from build123d import *

# Parameters (mm, degrees)
PAD029_DEPTH         = 16
SKETCH091_R          = 2.5
POCKET046_DEPTH      = 42.001
SKETCH092_R          = 2.63
POCKET047_DEPTH      = 30.001
POCKET047_DEPTH_BACK = 0.001


with BuildPart() as part:
    # Sketch089 → Pad029 (new body)
    with BuildSketch(Plane.XZ.offset(37.4)):
        with BuildLine():
            Line((-13, 31), (-10.5, 31))
            Line((-10.5, 10.5), (-10.5, 31))
            Line((10.5, 10.5), (-10.5, 10.5))
            Line((10.5, 31), (10.5, 10.5))
            Line((10.5, 31), (13, 31))
            ThreePointArc((15, 29), (14.414214, 30.414214), (13, 31))
            Line((15, 29), (15, 5.5))
            Line((15, 5.5), (13, 3.5))
            Line((13, 3.5), (13, -3.5))
            Line((13, -3.5), (15, -5.5))
            Line((15, -5.5), (15, -11))
            Line((15, -11), (-15, -11))
            Line((-15, -11), (-15, -5.5))
            Line((-13, -3.5), (-15, -5.5))
            Line((-13, 3.5), (-13, -3.5))
            Line((-15, 5.5), (-13, 3.5))
            Line((-15, 5.5), (-15, 29))
            ThreePointArc((-13, 31), (-14.414214, 30.414214), (-15, 29))
        make_face()
    extrude(amount=-PAD029_DEPTH)

    # Sketch091 → Pocket046 (cut, through all)
    with BuildSketch(Plane(origin=(0, 0, -11), x_dir=(-1, 0, 0), z_dir=(0, 0, -1))):
        with Locations((0, -29)):
            Circle(SKETCH091_R)
    extrude(amount=-POCKET046_DEPTH, mode=Mode.SUBTRACT)

    # Sketch092 → Pocket047 (cut, two sides)
    with BuildSketch(Plane(origin=(15, -29.4, 0), x_dir=(0, 1, 0), z_dir=(1, 0, 0))) as pocket047_sk:
        with Locations((0, 22)):
            Circle(SKETCH092_R)
    extrude(amount=-POCKET047_DEPTH, mode=Mode.SUBTRACT)
    extrude(pocket047_sk.sketch, amount=POCKET047_DEPTH_BACK, mode=Mode.SUBTRACT)


solid = part.part
CAD build for the part. Positions are in the model's coordinates, mm. A direction names the side the tool comes from. Coordinates: 2 decimals unless noted, no trailing zeros. Loops run counter-clockwise (first coordinate to the right, second up) from the corner with the lowest first, then second, coordinate; pieces in that order, holes last. Notation, with made-up numbers: (-29, -0.75) -> (-21, -0.75) arc R18 ccw to (-21, 8.25) -> close; hole circle Ø1 at (0.25, 55). An arc over 180 degrees is marked (long way). One line per item, written item: value.
1. Flat gauge pins, fed straight in: P1, Ø5.5, axis at y = -28, z = 1, coming from the -X side; P2, Ø5.5, axis at y = -26.5, z = 1, coming from the +X side; P3, Ø4.5, axis at y = -29.4, z = 22, coming from the +X side; P4, Ø6.5, axis at x = 0, y = -29, coming from the +Z side. Where does each tip first touch, or does it go through?
Answers:
P1: stops at x = -13.25
P2: stops at x = 13.25
P3: passes through
P4: stops at z = 10.5
2. Slice it at D-D on z = 22. Write the cut outline in (x, y), and give its area (3 significant figures).
Answers:
outline: (-15, -37.4) -> (-10.5, -37.4) -> (-10.5, -32.03) -> (-15, -32.03) -> close; (-15, -26.77) -> (-10.5, -26.77) -> (-10.5, -21.4) -> (-15, -21.4) -> close; (10.5, -37.4) -> (15, -37.4) -> (15, -32.03) -> (10.5, -32.03) -> close; (10.5, -26.77) -> (15, -26.77) -> (15, -21.4) -> (10.5, -21.4) -> close
area: 96.7 mm^2
3. Which spindle directions (+Z, -Z, +X, -X, +Y, -Y) get a long thin tool onto all of the face, cutting with end or side? Do faces 1 (the face through (-10.5, -30, 18)), 2 (the face through (-14, -29.5, -4.5)), 3 (the face through (13, -30, 0)), 4 (the face through (15, -30, -8)), 5 (the face through (-14.4, -29.51, 30.43)). Say none if no direction does.
Answers:
face 1: +Z, +Y, -Y
face 2: -X, +Y, -Y
face 3: +X, +Y, -Y
face 4: +Z, -Z, +X, +Y, -Y
face 5: +Z, -X, +Y, -Y
4. Slice it at A-A on z = 17.5. Write the cut outline in (x, y), and give its area (3 significant figures).
Answers:
outline: (-15, -37.4) -> (-10.5, -37.4) -> (-10.5, -21.4) -> (-15, -21.4) -> close; (10.5, -37.4) -> (15, -37.4) -> (15, -21.4) -> (10.5, -21.4) -> close
area: 144 mm^2
5. Pull direction Y, two halves, no side cores. Call faces 6 (the face through (-12, -30, 31)), 7 (the face through (0, -37.4, 6)), 8 (the face through (0.33, -26.52, -0.4)): pulls with the +Y half, pulls with the -Y half, needs draft (parallel to the pull), parting line crosses it, or undercut.
Answers:
face 6: needs draft
face 7: pulls with the -Y half
face 8: undercut
6. Drill centre lines: line 1 (X direction, y = -33.25, z = 14.5); line 2 (Z direction, x = 13.3, y = -29.4); line 3 (Y direction, x = 0, z = -3). Where is each one in solid material? Low to high. Write a range as [from, to].
Answers:
line 1: x = [-15, -10.5], [10.5, 15]
line 2: z = [-11, -3.8], [3.8, 19.37], [24.63, 30.98]
line 3: y = [-37.4, -31.5], [-26.5, -21.4]
7. Slice it at C-C on y = -29. Give the number of separate pieces and of enclosed holes in the cut face, and give its area (3 significant figures).
Answers:
separate pieces: 4
enclosed holes: 0
area: 637 mm^2
8. Slice it at B-B on x = 0. Write the cut outline in (y, z), and give its area (4 significant figures).
Answers:
outline: (-37.4, -11) -> (-31.5, -11) -> (-31.5, 10.5) -> (-37.4, 10.5) -> close; (-26.5, -11) -> (-21.4, -11) -> (-21.4, 10.5) -> (-26.5, 10.5) -> close
area: 236.5 mm^2
